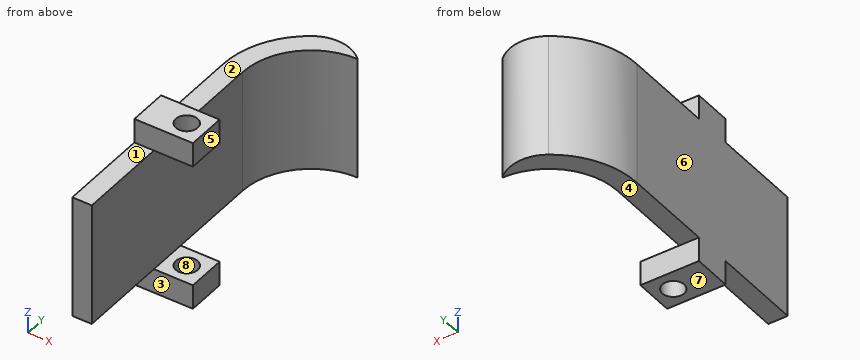
```python
from build123d import *

# Parameters (mm, degrees)
SURFACE_EXTRUDE2_1_DEPTH = 16.002
THICKEN2_T1              = 2.54
FILLET3_R                = 5.08
SURFACE_KNIT2_DEPTH      = 16.002
SKETCH6_R                = 1.4224
BOSS_EXTRUDE1_DEPTH      = 3.175


with BuildPart() as body_1:
    # Surface-Extrude2: a surface, the sketch's curves swept straight by 16.002 mm
    with BuildLine(Plane.XY, mode=Mode.PRIVATE) as surface_extrude2_1_path:
        Line((0, 0), (0, 28.702))
        ThreePointArc((0, 28.702), (2.603820715, 34.988179285), (8.89, 37.592))
    surface_extrude2_1 = Shell.extrude(surface_extrude2_1_path.wire(), (0 * SURFACE_EXTRUDE2_1_DEPTH, 0 * SURFACE_EXTRUDE2_1_DEPTH, 1 * SURFACE_EXTRUDE2_1_DEPTH))
    add(Solid.thicken(surface_extrude2_1, THICKEN2_T1))

    # Fillet3
    # the kernel refuses this fillet: 5.08 mm, written as the material it takes off along each edge
    with BuildSketch(Plane(origin=(8.89, 40.132, -16.731806751), x_dir=(-0.9561828874675108, -0.29277002188457374, 0), z_dir=(0, 0, 1))) as fillet3_piece_1:
        with BuildLine():
            CenterArc((5.205450989, 4.857409068), FILLET3_R, 208.560825218, 78.463040967)
            Line((0.743635856, 2.428704534), (0.654399553, 2.380130443))
            ThreePointArc((0.654399553, 2.380130443), (0.274669746, 1.244097701), (-0.097148181, 0.029745434))
            Line((-0.097148181, 0.029745434), (-0.029745434, -0.097148181))
            ThreePointArc((-0.029745434, -0.097148181), (3.34636135, -0.602429596), (6.722468135, -0.097148181))
            Line((6.722468135, -0.097148181), (6.6927227, 0))
        make_face()
    extrude(amount=49.465613501, mode=Mode.SUBTRACT)


with BuildPart() as body_2:
    # Surface-Knit2: read off the stored shape, not the designer's step
    # Surface-Knit2 outline → Surface-Knit2 (new body)
    with BuildSketch(Plane.XY):
        with BuildLine():
            Line((-2.54, 28.702), (-2.54, 0))
            Line((-2.54, 0), (0, 0))
            Line((0, 0), (0, 28.702))
            ThreePointArc((0, 28.702), (2.603820715, 34.988179285), (8.89, 37.592))
            ThreePointArc((8.89, 37.592), (5.793722616, 39.022651388), (2.490533083, 38.172571429))
            ThreePointArc((2.490533083, 38.172571429), (-1.204325308, 34.063855702), (-2.54, 28.702))
        make_face()
    extrude(amount=SURFACE_KNIT2_DEPTH)

    # Sketch6 → Boss-Extrude1 (add)
    with BuildSketch(Plane.XY.offset(16.002)):
        Polygon((0, 11.811), (5.08, 11.811), (5.08, 16.891), (0, 16.891), (-2.54, 16.891), (-2.54, 11.811), align=None)
        with Locations((2.54, 14.351)):
            Circle(SKETCH6_R, mode=Mode.SUBTRACT)
    boss_extrude1 = extrude(amount=BOSS_EXTRUDE1_DEPTH)

    # Mirror1: Boss-Extrude1 across plane
    add(boss_extrude1.mirror(Plane(origin=(0, 0, 8.001), x_dir=(1, 0, 0), z_dir=(0, 0, -1))))


solid = body_2.part
```
Build history of the part. All positions in model axes, mm. Face numbers are marked on the shaded views. A direction names the side the tool comes from. Round coordinates to 2 decimals unless told otherwise and drop trailing zeros. Order: outer loops, then holes, each group sorted by start corner. A loop starts at its lowest first (then second) coordinate and runs counter-clockwise, first axis right, second up. Notation, with made-up numbers: (65.25, -29) - (123.25, -29) arc R25 cw to (123.25, 6) - close; hole circle Ø8 at (33, 29). An arc over 180 degrees is marked (long way). Use a Markdown table: item, result.
1) Pull direction X, two halves, no side cores. Call the marked faces 5, 6, 7 and 8: pulls with the +X half, pulls with the -X half, needs draft (parallel to the pull), parting line crosses it, or undercut.
Recorded:
| item | result |
|---|---|
| face 5 | pulls with the +X half |
| face 6 | pulls with the -X half |
| face 7 | needs draft |
| face 8 | undercut |
2) Saw through at A-A on x = 3. Write the cut outline in (y, z) (3 decimals).
Recorded:
| item | result |
|---|---|
| outline | (11.811, -3.175) - (13.005, -3.175) - (13.005, 0) - (11.811, 0) - close; (11.811, 16.002) - (13.005, 16.002) - (13.005, 19.177) - (11.811, 19.177) - close; (15.697, -3.175) - (16.891, -3.175) - (16.891, 0) - (15.697, 0) - close; (15.697, 16.002) - (16.891, 16.002) - (16.891, 19.177) - (15.697, 19.177) - close; (35.361, 0) - (38.475, 0) - (38.475, 16.002) - (35.361, 16.002) - close |
3) Tool access for the marked faces 1, 2, 3 and 4: list every direction of +Z, -Z, +X, -X, +Y, -Y with a clear straight run to the whole face (end or side of a thin tool).
Recorded:
| item | result |
|---|---|
| face 1 | +Z, +X, -X, -Y |
| face 2 | +Z, +X, -X, +Y |
| face 3 | -Z, +X, -X, -Y |
| face 4 | -Z, +X, -X, +Y |
4) Saw through at B-B on y = 12.5. Write the cut outline in (x, z) (3 decimals), and give its area (3 significant figures).
Recorded:
| item | result |
|---|---|
| outline | (-2.54, -3.175) - (5.08, -3.175) - (5.08, 0) - (0, 0) - (0, 16.002) - (5.08, 16.002) - (5.08, 19.177) - (-2.54, 19.177) - close |
| area | 89.0 mm² |
5) Saw through at C-C on z = 4.25. Write the cut outline in (x, y).
Recorded:
| item | result |
|---|---|
| outline | (-2.54, 0) - (0, 0) - (0, 28.7) arc R8.89 cw to (8.89, 37.59) arc R5.08 ccw to (2.49, 38.17) arc R11.43 ccw to (-2.54, 28.7) - close |
6) Wall check: L1, parallel to Y at x = 2.54, z = 17.05; L2, parallel to Y at x = 0.5, z = 16.25; L3, parallel to X at y = 8.5, z = 3.75. Give the ranges that are in metal, low to high.
Recorded:
| item | result |
|---|---|
| L1 | y = 11.81 to 12.93, 15.77 to 16.89 |
| L2 | y = 11.81 to 16.89 |
| L3 | x = -2.54 to 0 |
7) Flat gauge pins, fed straight in: pin 1 Ø0.8 at (x, y) = (-1, 6.5) entering from +Z; pin 2 Ø3.5 at (y, z) = (15, -2) entering from +X; pin 3 Ø1 at (x, z) = (1, 18) entering from -Y. Where does each tip first touch, or does it go through?
Recorded:
| item | result |
|---|---|
| pin 1 | stops at z = 16 |
| pin 2 | stops at x = 5.08 |
| pin 3 | stops at y = 11.81 |
8) Saw through at D-D on x = -1.25. Write the cut outline in (y, z) (3 decimals), and give its area (3 significant figures).
Recorded:
| item | result |
|---|---|
| outline | (0, 0) - (11.811, 0) - (11.811, -3.175) - (16.891, -3.175) - (16.891, 0) - (33.977, 0) - (33.977, 16.002) - (16.891, 16.002) - (16.891, 19.177) - (11.811, 19.177) - (11.811, 16.002) - (0, 16.002) - close |
| area | 576 mm² |
